Can you work these out from the drawing? Everything is in mm from the part's minimum corner. A direction names the side the tool comes from. Coordinates: 2 decimals unless noted, no trailing zeros. Order: outer loops, then holes, each group sorted by start corner. A loop starts at its lowest first (then second) coordinate and runs counter-clockwise, first axis right, second up. Notation, with made-up numbers: (15, 14.5) - (56, 14.5) arc R14 ccw to (56, 29.5) - close; hole circle Ø9 at (-16, -31). An arc over 180 degrees is marked (long way). One line per item, written item: value.
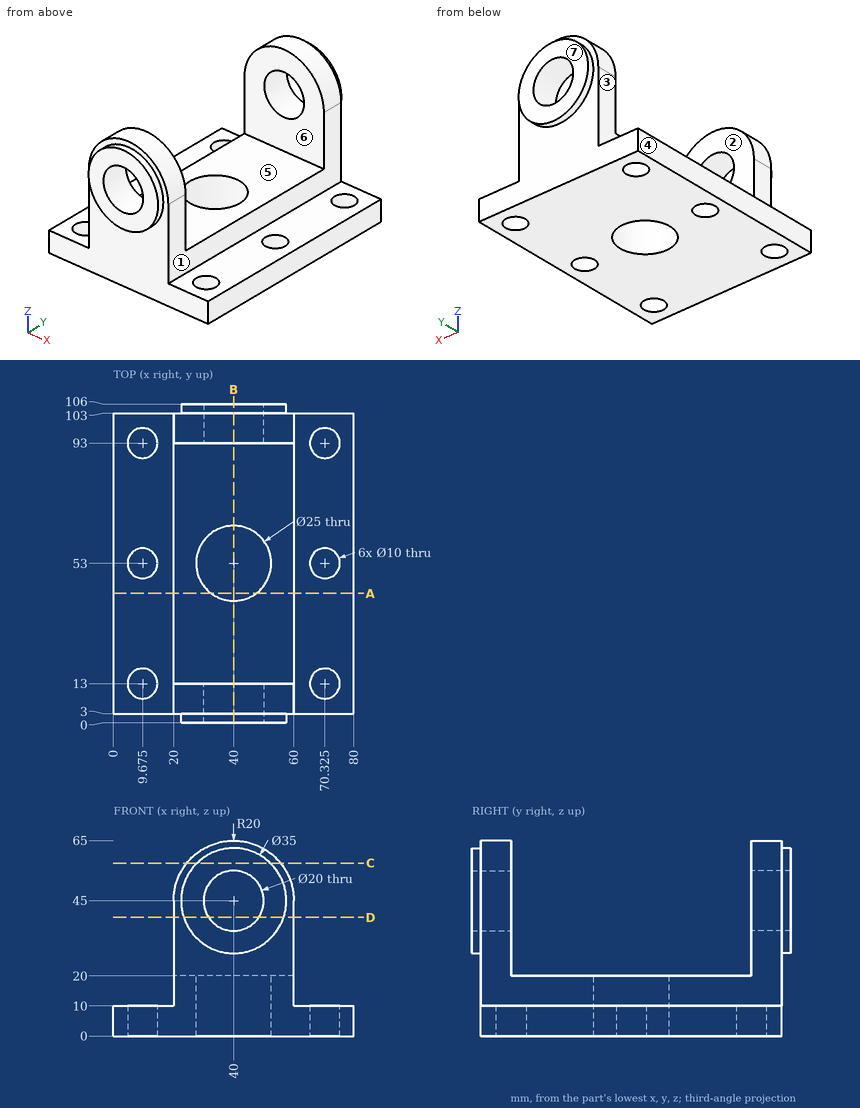
Item 1: I want a section at D-D on z = 39.5. Please give me the cut outline in (x, y), then the cut area to 3 significant figures.
Conclusion:
outline: (20, 3) - (23.39, 3) - (23.39, 0) - (31.65, 0) - (31.65, 13) - (20, 13) - close; (20, 93) - (31.65, 93) - (31.65, 106) - (23.39, 106) - (23.39, 103) - (20, 103) - close; (48.35, 0) - (56.61, 0) - (56.61, 3) - (60, 3) - (60, 13) - (48.35, 13) - close; (48.35, 93) - (60, 93) - (60, 103) - (56.61, 103) - (56.61, 106) - (48.35, 106) - close
area: 565 mm²
Item 2: I want a section at C-C on z = 57.5. Please give me the cut outline in (x, y).
Conclusion:
outline: (24.39, 3) - (27.75, 3) - (27.75, 0) - (52.25, 0) - (52.25, 3) - (55.61, 3) - (55.61, 13) - (24.39, 13) - close; (24.39, 93) - (55.61, 93) - (55.61, 103) - (52.25, 103) - (52.25, 106) - (27.75, 106) - (27.75, 103) - (24.39, 103) - close
Item 3: If I drill on probe 1 along Y at (x, z) = (55, 52); probe 2 along Z at (x, y) = (40, 6.75); probe 3 along X at (y, z) = (92, 4), over which ranges is the centre line in solid material (lowest first)?
Conclusion:
probe 1: 0 to 13, 93 to 106
probe 2: 0 to 35, 55 to 65
probe 3: 0 to 4.78, 14.57 to 65.43, 75.22 to 80
Item 4: For the marked faces 1, 2 and 3, which set-ups out of +Z, -Z, +X, -X, +Y, -Y let a thin tool reach every point of the face, with its end or its side?
Conclusion:
face 1: +Z, +X, +Y, -Y
face 2: +Z, +X, -X
face 3: +Z, -X, +Y, -Y
Item 5: I want a section at B-B on x = 40. Please give me the cut outline in (y, z).
Conclusion:
outline: (0, 27.5) - (3, 27.5) - (3, 0) - (40.5, 0) - (40.5, 20) - (13, 20) - (13, 35) - (0, 35) - close; (0, 55) - (13, 55) - (13, 65) - (3, 65) - (3, 62.5) - (0, 62.5) - close; (65.5, 0) - (103, 0) - (103, 27.5) - (106, 27.5) - (106, 35) - (93, 35) - (93, 20) - (65.5, 20) - close; (93, 55) - (106, 55) - (106, 62.5) - (103, 62.5) - (103, 65) - (93, 65) - close
Item 6: Thinking about a two-plate mould opening in Y: for the marked faces 4, 5, 6 and 7, which applies, pulls with the +Y half, pulls with the -Y half, needs draft (parallel to the pull), parting line crosses it, or undercut?
Conclusion:
face 4: needs draft
face 5: undercut
face 6: undercut
face 7: pulls with the +Y half
Item 7: I'm going to push flat-ended pins straight in: pin 1 Ø2 at (x, z) = (55.5, 24) entering from -Y; pin 2 Ø16 at (x, y) = (9.675, 93) entering from +Z; pin 3 Ø3 at (x, z) = (61, 46.5) entering from +Y. Where does each tip first touch, or does it pass through?
Conclusion:
pin 1: y = 3
pin 2: z = 10
pin 3: y = 103
Item 8: I want a section at A-A on y = 43. Please give me the cut outline in (x, z), then the cut area to 3 significant figures.
Conclusion:
outline: (0, 0) - (32.5, 0) - (32.5, 20) - (20, 20) - (20, 10) - (0, 10) - close; (47.5, 0) - (80, 0) - (80, 10) - (60, 10) - (60, 20) - (47.5, 20) - close
area: 900 mm²
